Can you work these out from the drawing? Everything is in mm from the part's minimum corner. Give positions to 0.01 mm unless a question says otherwise; leave off trailing zeros. Write each loop counter-clockwise with the first axis right and the second up, starting at its lowest first coordinate (ties: lowest second). Pieces come first, ordered by that corner, then holes. Notation, with made-up numbers: (-15.5, -28) -> (37.5, -28) arc R18 ccw to (37.5, 6) -> close; hole circle Ø10 at (43, -34.75). An arc over 180 degrees is marked (long way). Answer as CSV lines item,"result". Start each with the question number.
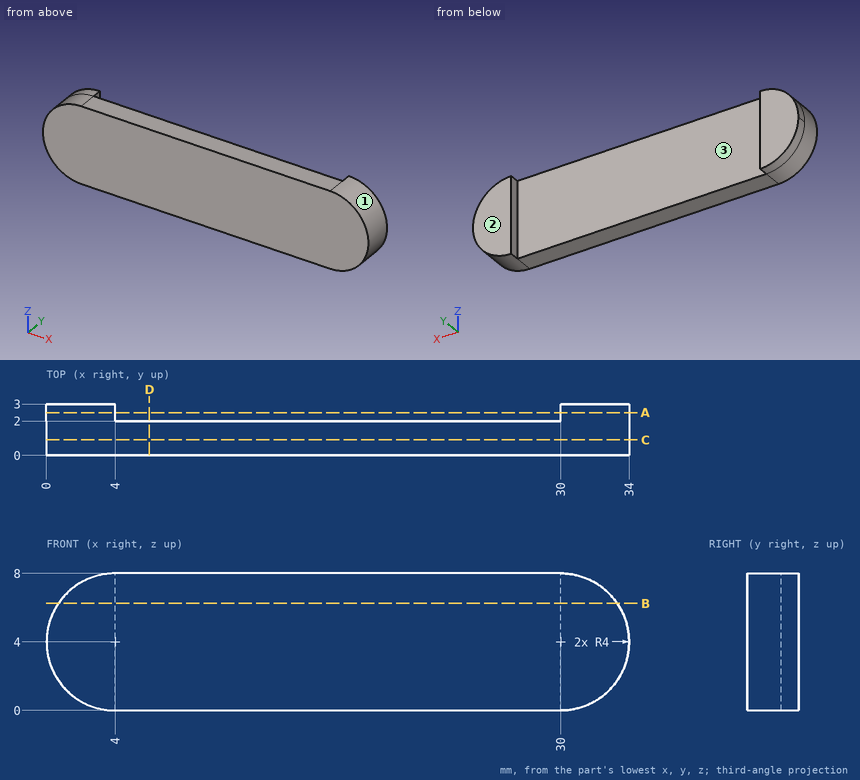
Item 1: I'm going to push a flat-ended pin straight in: pin 1 (4 mm diameter, centred on x = 15.5, z = 5, fed in from +Y). Where does the tip first touch, or does it pass through?
Item 2: We'd pull the mould along X, two halves only. Please class the marked faces 1, 2 and 3: released by +X, released by -X, zero draft, split by the parting line, or undercut.
Item 3: If we section it at C-C (y = 0.9): Please give me the cut outline in (x, z).
Item 4: If we section it at B-B (z = 6.25): Please give me the cut outline in (x, y), and give its area (3 significant figures).
Item 5: If we section it at A-A (y = 2.5): Please give me the cut outline in (x, z), and give its area (3 significant figures).
Item 6: If we section it at D-D (x = 6): Please give me the cut outline in (y, z).
Item 7: If I drill on line 1 (Y direction, x = 16.5, z = 2.75); line 2 (X direction, y = 2.65, z = 1); line 3 (X direction, y = 0.35, z = 5.5), over which ranges is the centre line in solid material (lowest first)? Write a range as [from, to].
Final values:
1,pin 1,"y = 2"
2,face 1,"released by +X"
2,face 2,"zero draft"
2,face 3,"undercut"
3,outline,"(4, 0) -> (30, 0) arc R4 ccw to (30, 8) -> (4, 8) arc R4 ccw to start"
4,outline,"(0.69, 0) -> (33.31, 0) -> (33.31, 3) -> (30, 3) -> (30, 2) -> (4, 2) -> (4, 3) -> (0.69, 3) -> close"
4,area,"71.8 mm2"
5,outline,"(4, 0) -> (4, 8) arc R4 ccw to start; (30, 0) arc R4 ccw to (30, 8) -> close"
5,area,"50.3 mm2"
6,outline,"(0, 0) -> (2, 0) -> (2, 8) -> (0, 8) -> close"
7,line 1,"[0, 2]"
7,line 2,"[1.35, 4], [30, 32.65]"
7,line 3,"[0.29, 33.71]"
